For this review, take the finished solid that the model builds, in its own axes (mm). A direction names the side the tool comes from. Coordinates: 2 decimals unless noted, no trailing zeros. Loops run counter-clockwise (first coordinate to the right, second up) from the corner with the lowest first, then second, coordinate; pieces in that order, holes last.
1. Take a section at C-C, the plane x = -63.5. State the section outline as (y, z) points.
2. To check wall thickness, follow probe 1 along Z at (x, y) = (-55.75, 66.5); probe 2 along Z at (x, y) = (-57.25, 56.75); probe 3 along Z at (x, y) = (-60.25, 51). State the ranges of each line that lie inside material, in increasing order.
3. Take a section at B-B, the plane y = 66. State the section outline as (x, z) points.
4. Mouldability with a two-part tool opening along Z and no side actions: class faces 4 (the face through (-64, 52, 0)), 5 (the face through (-58.449, 66.665, 19.314)), 6 (the face through (-56, 49.13, 2)) as pulls with the +Z half, pulls with the -Z half, needs draft (parallel to the pull), parting line crosses it, or undercut.
5. Machinability: for faces 1 (the face through (-56, 59, 0)), 2 (the face through (-56, 64.13, 24)), 3 (the face through (-64, 67, 0)), which of the approach directions +Z, -Z, +X, -X, +Y, -Y give a long, thin tool a straight path to every point of the face, cutting with its end or side? Answer none if there is none.
6. Take a section at D-D, the plane z = -107.5. State the section outline as (x, y) points, then the cut area to 3 significant figures.
7. Clearance check with flat-ended pins moving along their axes: P1, Ø8, axis at y = 67, z = -101.5, coming from the -X side; P2, Ø1, axis at x = -51.5, z = -36, coming from the -Y side; P3, Ø8, axis at x = -52, y = 53, coming from the +Z side. State where each tip first meets the part, or that it passes through.
8. Take a section at A-A, the plane z = 23.75. State the section outline as (x, y) points.
```python
from build123d import *

# Parameters (mm, degrees)
F0_W     = 20
F0_H     = 20
F1_DEPTH = 5
F2_R     = 3.75
F3_DEPTH = 150
F4_W     = 20
F4_H     = 10
F5_DEPTH = 30
F6_R     = 5
F7_DEPTH = 5


with BuildPart() as f1:
    # F0 (on Top) → F1 (new body)
    with BuildSketch(Plane.XY):
        with Locations((-56.141918, 59.129702)):
            Rectangle(F0_W, F0_H)
    extrude(amount=F1_DEPTH)

    # F2 (on face) → F3 (join)
    with BuildSketch(Plane(origin=(0, 0, 0), x_dir=(1, 0, 0), z_dir=(0, 0, -1))):
        with BuildLine():
            ThreePointArc((-56.141918, -69.129702), (-49.07085, -66.20077), (-46.141918, -59.129702))
            ThreePointArc((-46.141918, -59.129702), (-49.07085, -52.058634), (-56.141918, -49.129702))
            ThreePointArc((-56.141918, -49.129702), (-63.212986, -52.058634), (-66.141918, -59.129702))
            ThreePointArc((-66.141918, -59.129702), (-63.212986, -66.20077), (-56.141918, -69.129702))
        make_face()
        with Locations((-56.141918, -59.129702)):
            Circle(F2_R, mode=Mode.SUBTRACT)
    extrude(amount=F3_DEPTH)

    # F4 (on face) → F5 (join)
    with BuildSketch(Plane.XY.offset(5)):
        with Locations((-56.141918, 64.129702)):
            Rectangle(F4_W, F4_H)
    extrude(amount=F5_DEPTH)

    # F6 (on face) → F7 (cut)
    with BuildSketch(Plane(origin=(0, 69.129702, 0), x_dir=(-1, 0, 0), z_dir=(0, 1, 0))):
        with Locations((56.141918, 23.75)):
            Circle(F6_R)
    extrude(amount=-F7_DEPTH, mode=Mode.SUBTRACT)


solid = f1.part
```
Results list:
1. outline: (49.13, 0) - (52.36, 0) - (52.36, -150) - (65.9, -150) - (65.9, 0) - (69.13, 0) - (69.13, 35) - (59.13, 35) - (59.13, 5) - (49.13, 5) - close
2. probe 1: z = -150 to 18.77, 28.73 to 35
2. probe 2: z = 0 to 5
2. probe 3: z = -150 to 5
3. outline: (-66.14, 0) - (-63.41, 0) - (-63.41, -150) - (-48.88, -150) - (-48.88, 0) - (-46.14, 0) - (-46.14, 35) - (-66.14, 35) - close; hole circle Ø10 at (-56.14, 23.75)
4. face 4: pulls with the -Z half
4. face 5: undercut
4. face 6: needs draft
5. face 1: -Z
5. face 2: +Y
5. face 3: -Z, -X, +Y
6. outline: (-66.14, 59.13) arc R10 ccw to (-56.14, 49.13) arc R10 ccw to (-46.14, 59.13) arc R10 ccw to (-56.14, 69.13) arc R10 ccw to start; hole circle Ø7.5 at (-56.14, 59.13)
6. area: 270 mm2
7. P1: stops at x = -65.36
7. P2: stops at y = 50.03
7. P3: stops at z = 5
8. outline: (-66.14, 59.13) - (-46.14, 59.13) - (-46.14, 69.13) - (-51.14, 69.13) - (-51.14, 64.13) - (-61.14, 64.13) - (-61.14, 69.13) - (-66.14, 69.13) - close
